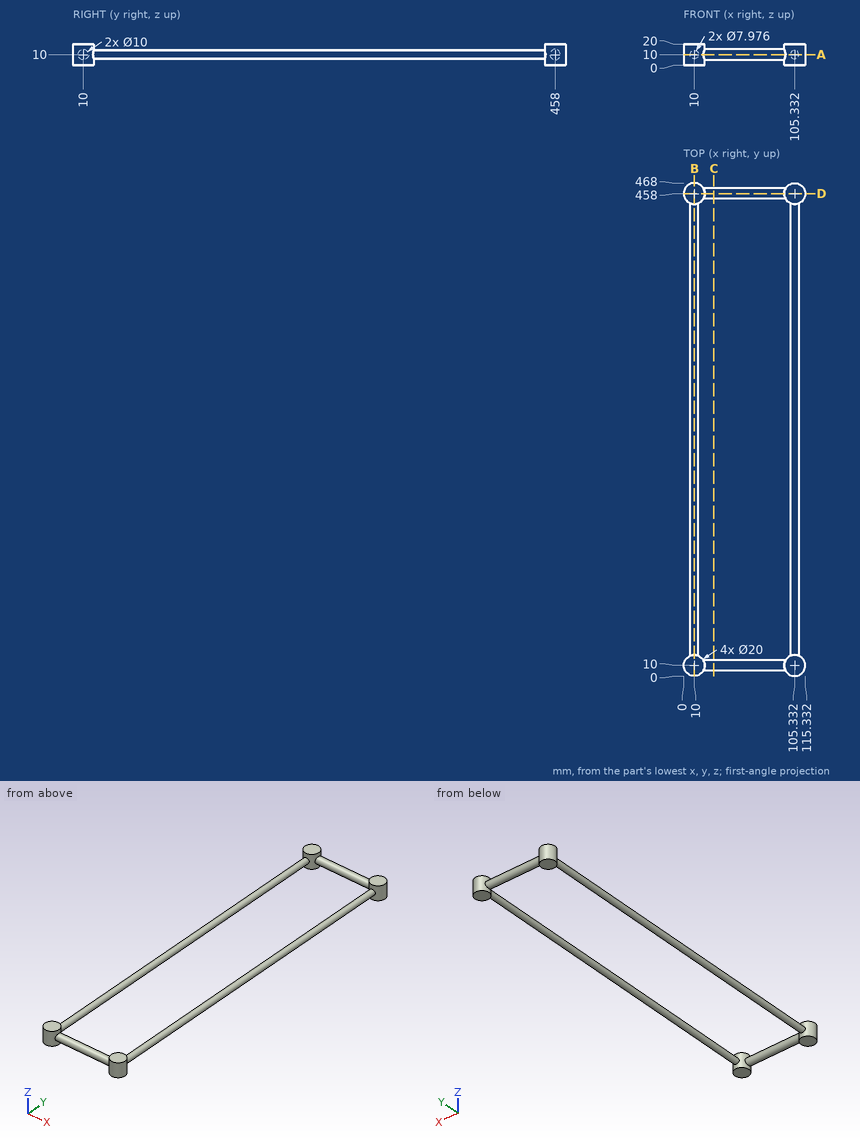
Geometry: see drawing. Coordinates: mm, zero at the bounding-box minimum. Round coordinates to 2 decimals unless told otherwise and drop trailing zeros. Loops run counter-clockwise (first coordinate to the right, second up) from the corner with the lowest first, then second, coordinate; pieces in that order, holes last. Notation, with made-up numbers: M 1.5,32.5 L 14.5,32.5 A35 cw 14.5,68.5 Z; hole C 88,17.5 d6. An arc over 180 degrees is marked long. Use a Markdown table: item, result. Add a question column.
1. Contact query for flat-ended pins moving along their axis: P1, Ø12, axis at x = 94.5, z = 6.5, coming from the -Y side (1 decimal); P2, Ø5, axis at y = 357.5, z = 17, coming from the +X side; P3, Ø3, axis at x = 39, z = 15, coming from the +Y side; P4, Ø10, axis at x = 17, y = 316, coming from the +Z side. Output: stop coordinate, or through.
2. Section query C-C on x = 28.5. Return the cut outline in (y, z).
3. Section query B-B on x = 10. Return the cut outline in (y, z).
4. Line query: line 1 (X direction, y = 66, z = 9.5) (1 decimal); line 2 (X direction, y = 130, z = 13) (1 decimal); line 3 (Y direction, x = 49, z = 7). Output: solid intervals per line, ascending.
5. Section query D-D on y = 458. Return the cut outline in (x, z), then the cut area to 3 significant figures.
6. Section query A-A on z = 10. Return the cut outline in (x, y), then the cut area to 3 significant figures.
Reported:
| question | item | result |
|---|---|---|
| 1 | P1 | stops at y = 1.2 |
| 1 | P2 | passes through |
| 1 | P3 | stops at y = 461.57 |
| 1 | P4 | stops at z = 13.45 |
| 2 | outline | C 10,10 d10; C 458,10 d10 |
| 3 | outline | M 0,0 L 20,0 L 20,6.01 L 448,6.01 L 448,0 L 468,0 L 468,20 L 448,20 L 448,13.99 L 20,13.99 L 20,20 L 0,20 Z |
| 4 | line 1 | x = 6 to 14, 101.4 to 109.3 |
| 4 | line 2 | x = 7.4 to 12.6, 102.7 to 108 |
| 4 | line 3 | y = 6 to 14, 454 to 462 |
| 5 | outline | M 0,0 L 20,0 L 20,5 L 95.33,5 L 95.33,0 L 115.33,0 L 115.33,20 L 95.33,20 L 95.33,15 L 20,15 L 20,20 L 0,20 Z |
| 5 | area | 1,550 mm² |
| 6 | outline | M 6.01,19.17 A10 ccw long 18.66,5 L 96.67,5 A10 ccw long 109.32,19.17 L 109.32,448.83 A10 ccw long 96.67,463 L 18.66,463 A10 ccw long 6.01,448.83 Z; hole M 13.99,19.17 A10 cw 18.66,15 L 96.67,15 A10 cw 101.34,19.17 L 101.34,448.83 A10 cw 96.67,453 L 18.66,453 A10 cw 13.99,448.83 Z |
| 6 | area | 9,620 mm² |
